from build123d import *

# Parameters (mm, degrees)
F0_R     = 1.5
F1_DEPTH = 8
F2_W     = 30.229195
F2_H     = 14.570514
F3_DEPTH = 25.4
F4_W     = 10.16
F4_H     = 6.534409
F5_DEPTH = 25.4


with BuildPart() as f1:
    # F0 (on Front) → F1 (new body, symmetric)
    with BuildSketch(Plane.XZ):
        with BuildLine():
            Line((9.825, 3.5), (-9.825, 3.5))
            ThreePointArc((-9.825, 3.5), (-13.325, 0), (-9.825, -3.5))
            Line((-9.825, -3.5), (9.825, -3.5))
            ThreePointArc((9.825, -3.5), (13.325, 0), (9.825, 3.5))
        make_face()
        with Locations((-9.825, 0)):
            Circle(F0_R, mode=Mode.SUBTRACT)
        with Locations((9.825, 0)):
            Circle(F0_R, mode=Mode.SUBTRACT)
    extrude(amount=F1_DEPTH, both=True)

    # F2 (on face) → F3 (cut)
    with BuildSketch(Plane.XY.offset(3.5)):
        with Locations((10.034598, -7.635257)):
            Rectangle(F2_W, F2_H)
    extrude(amount=-F3_DEPTH, mode=Mode.SUBTRACT)

    # F4 (on face) → F5 (cut)
    with BuildSketch(Plane.XZ.offset(0.35)):
        with Locations((0, 3.267205)):
            Rectangle(F4_W, F4_H)
    extrude(amount=-F5_DEPTH, mode=Mode.SUBTRACT)


solid = f1.part
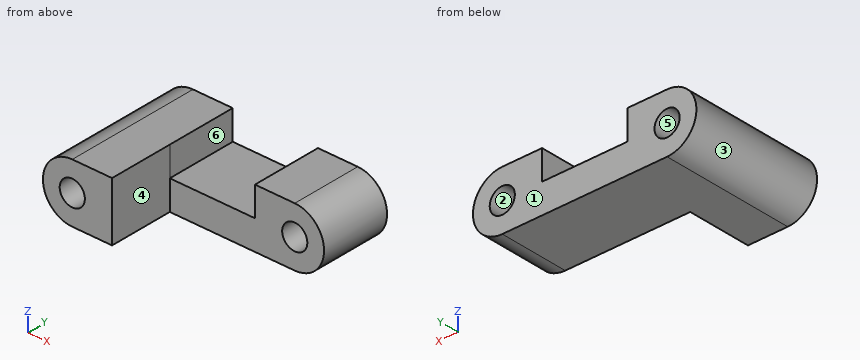
Could you check a few things on this model? Use its own coordinates, in mm. Face numbers are marked on the shaded views. A direction names the side the tool comes from. Give positions to 0.01 mm unless a question says otherwise; leave off trailing zeros. Order: outer loops, then holes, each group sorted by start corner. A loop starts at its lowest first (then second) coordinate and runs counter-clockwise, first axis right, second up. Notation, with made-up numbers: (62, 20.25) - (105, 20.25) arc R31 cw to (105, 49.25) - close; hole circle Ø3 at (-9.5, 58). An arc over 180 degrees is marked (long way). Return JSON: item names as keys, results as strings. Group by question number.
Q1. Suppose I cut it at C-C, the plane x = 10.25. Please give me the cut outline in (y, z).
Q2. Suppose I cut it at D-D, the plane z = -0.75. Please give me the cut outline in (x, y), and give its area (3 significant figures).
Q3. Will these pins go through, and if not, where does the flat tip stop? pin 1 Ø2 at (y, z) = (-5.5, 0.5) entering from +X; pin 2 Ø1 at (y, z) = (5, 1) entering from +X; pin 3 Ø1 at (y, z) = (5, 1) entering from -X.
Q4. Please list where these lines run through material, in increasing order: line 1 along X through (y, z) = (0, 1); line 2 along X through (y, z) = (5.75, -0.25); line 3 along X through (y, z) = (6.25, -0.75). Write a range as [from, to].
Q5. Suppose I cut it at A-A, the plane y = 6. Please give me the cut outline in (x, z) (3 decimals), and give its area (3 significant figures).
Q6. Which directions (+Z, -Z, +X, -X, +Y, -Y) give clear straight access to the entire face, cutting with the end or side of a thin tool? Please do the marked faces 4, 5 and 6.
Q7. Thinking about a two-plate mould opening in X: for the marked faces 1, 2 and 3, which applies, pulls with the +X half, pulls with the -X half, needs draft (parallel to the pull), parting line crosses it, or undercut?
Q8. Suppose I cut it at B-B, the plane z = 0.75. Please give me the cut outline in (x, y).
Resolved:
{
 "1": {"outline": "(-0.35, -3.47) - (8, -3.47) - (8, -1.44) - (-0.35, -1.44) - close; (-0.35, 1.44) - (8, 1.44) - (8, 3.47) - (-0.35, 3.47) - close"},
 "2": {"outline": "(-13.24, -8) - (-11.12, -8) - (-11.12, 8) - (-13.24, 8) - close; (-8.53, -8) - (-5.08, -8) - (-5.08, -0.35) - (8.53, -0.35) - (8.53, 8) - (-8.53, 8) - close; (11.12, -0.35) - (13.24, -0.35) - (13.24, 8) - (11.12, 8) - close", "area": "220 mm2"},
 "3": {"pin 1": "stops at x = -5.08", "pin 2": "stops at x = 13.29", "pin 3": "stops at x = -13.29"},
 "4": {"line 1": "x = [-13.18, -10.94], [-8.71, -5.08], [5.08, 8.71], [10.94, 13.18]", "line 2": "x = [-13.32, -11.3], [-8.35, 8.35], [11.3, 13.32]", "line 3": "x = [-13.24, -11.12], [-8.53, 8.53], [11.12, 13.24]"},
 "5": {"outline": "(-9.825, -3.5) - (9.825, -3.5) arc R3.5 ccw to (9.825, 3.5) - (5.08, 3.5) - (5.08, 0) - (-5.08, 0) - (-5.08, 3.5) - (-9.825, 3.5) arc R3.5 ccw to start; hole circle Ø3 at (-9.825, 0); hole circle Ø3 at (9.825, 0)", "area": "126 mm2"},
 "6": {"face 4": "+Z, -Z, +X, -Y", "face 5": "+Y, -Y", "face 6": "+Z, +Y, -Y"},
 "7": {"face 1": "needs draft", "face 2": "undercut", "face 3": "pulls with the -X half"},
 "8": {"outline": "(-13.24, -8) - (-11.12, -8) - (-11.12, 8) - (-13.24, 8) - close; (-8.53, -8) - (-5.08, -8) - (-5.08, 8) - (-8.53, 8) - close; (5.08, -0.35) - (8.53, -0.35) - (8.53, 8) - (5.08, 8) - close; (11.12, -0.35) - (13.24, -0.35) - (13.24, 8) - (11.12, 8) - close"}
}
